from build123d import *

# Parameters (mm, degrees)
BOSS_EXTRUDE2_DEPTH = 20
SKETCH2_R           = 1.025
SKETCH2_R_2         = 1.05
SKETCH2_R_3         = 0.975
SKETCH2_R_4         = 1
SKETCH2_R_5         = 2.5
SKETCH2_R_6         = 2.55
SKETCH2_R_7         = 2.525
BOSS_EXTRUDE3_DEPTH = 20


with BuildPart() as part:
    # Sketch1 → Boss-Extrude2 (new body)
    with BuildSketch(Plane(origin=(0, 0, 0), x_dir=(1, 0, 0), z_dir=(0, 1, 0))):
        Polygon((21, -13.279056191), (21, -19.052558883), (23, -19.052558883), (23, -13.279056191), (33, -7.505553499), (43, -13.279056191), (43, -19.052558883), (45, -19.052558883), (45, -13.279056191), (55, -7.505553499), (65, -13.279056191), (65, -19.052558883), (66, -19.052558883), (66, -11.547005384), (56, -5.773502692), (56, 5.773502692), (66, 11.547005384), (66, 26.452994616), (56, 32.226497308), (56, 38), (54, 38), (54, 32.226497308), (44, 26.452994616), (34, 32.226497308), (34, 38), (32, 38), (32, 32.226497308), (22, 26.452994616), (12, 32.226497308), (12, 38), (11, 38), (11, 30.494446501), (21, 24.720943809), (21, 13.173938425), (11, 7.400435733), (11, -7.505553499), align=None)
        Polygon((12, 5.773502692), (22, 11.547005384), (32, 5.773502692), (32, -5.773502692), (22, -11.547005384), (12, -5.773502692), align=None, mode=Mode.SUBTRACT)
        Polygon((34, 5.773502692), (44, 11.547005384), (54, 5.773502692), (54, -5.773502692), (44, -11.547005384), (34, -5.773502692), align=None, mode=Mode.SUBTRACT)
        Polygon((43, 13.173938425), (33, 7.400435733), (23, 13.173938425), (23, 24.720943809), (33, 30.494446501), (43, 24.720943809), align=None, mode=Mode.SUBTRACT)
        Polygon((65, 13.173938425), (55, 7.400435733), (45, 13.173938425), (45, 24.720943809), (55, 30.494446501), (65, 24.720943809), align=None, mode=Mode.SUBTRACT)
    extrude(amount=BOSS_EXTRUDE2_DEPTH)

    # Sketch2 → Boss-Extrude3 (add, through all)
    with BuildSketch(Plane(origin=(0, 20, 0), x_dir=(1, 0, 0), z_dir=(0, 1, 0))):
        Polygon((44, 11.547005384), (34, 5.773502692), (34, -5.773502692), (44, -11.547005384), (54, -5.773502692), (54, 5.773502692), align=None)
        with Locations((44, 7.57813322)):
            Circle(SKETCH2_R, mode=Mode.SUBTRACT)
        with Locations((49.12400919, 6.50535)):
            Circle(SKETCH2_R_2, mode=Mode.SUBTRACT)
        with Locations((49.12400919, 1.82801516)):
            Circle(SKETCH2_R_3, mode=Mode.SUBTRACT)
        with Locations((38.868201604, 4.488517546)):
            Circle(SKETCH2_R_4, mode=Mode.SUBTRACT)
        with Locations((38.567822302, -1.561979816)):
            Circle(SKETCH2_R_5, mode=Mode.SUBTRACT)
        with Locations((45.13325561, -4.136659545)):
            Circle(SKETCH2_R_6, mode=Mode.SUBTRACT)
        with Locations((51.012107657, -2.763497023)):
            Circle(SKETCH2_R_7, mode=Mode.SUBTRACT)
    extrude(amount=-BOSS_EXTRUDE3_DEPTH)


solid = part.part
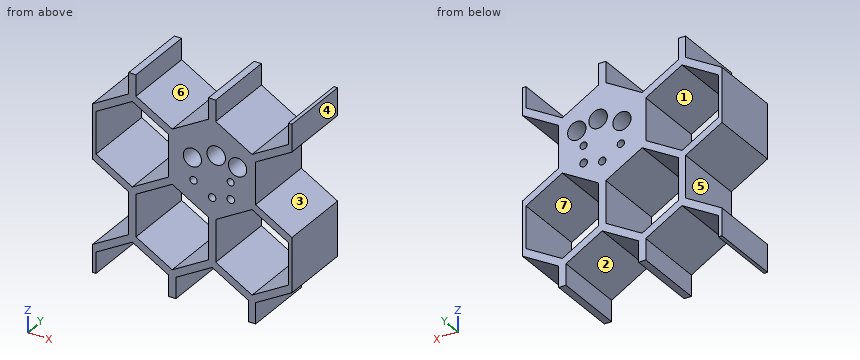
Source: CAD feature listing. Evaluate the final solid. Frame: model axes, mm. Face numbers are marked on the shaded views. A direction names the side the tool comes from. Round coordinates to 2 decimals unless told otherwise and drop trailing zeros. Loops run counter-clockwise (first coordinate to the right, second up) from the corner with the lowest first, then second, coordinate; pieces in that order, holes last. Notation, with made-up numbers: (-23, 50) - (-10, 50) arc R9 ccw to (-10, 64) - close; hole circle Ø6 at (34, 9). An arc over 180 degrees is marked (long way). Write item = value, one per line. Start each with the question number.
(1) Pin query (flat end, axial travel): pin 1 (6 mm diameter, centred on x = 33, z = -6.5, fed in from -Y); pin 2 (1 mm diameter, centred on x = 47.5, y = 13, fed in from +Z); pin 3 (1.7 mm diameter, centred on y = 13, z = 15, fed in from -X); pin 4 (6.5 mm diameter, centred on y = 14, z = -34, fed in from +X). Return the tip coordinate at first contact, or that it passes through.
(2) Section query C-C, the plane z = -10.5. Output: boundary loops of the cut face in (x, y).
(3) Set-up query: the marked faces 1, 2 and 3. Return all of +Z, -Z, +X, -X, +Y, -Y with unobstructed straight access to the full face (end or side cutting, diameter ignored); none if empty.
(4) Ray query, line 1 along X through (y, z) = (9.75, -24.5); line 2 along Z through (x, y) = (57.5, 16.25); line 3 along Z through (x, y) = (30, 8.5). Return the intervals inside material, ascending. Write a range as from..to.
(5) Section query D-D, the plane y = 2.5. State how many separate pieces and enclosed holes the cut face has, plus the area to 3 significant figures.
(6) Pull-direction query (Z, two-part tool) for the marked faces 4, 5, 6 and 7; classes: +Z half, -Z half, draft (parallel to the pull), parting line (faces both ways), or undercut.
(7) Section query B-B, the plane x = 29.5. Output: boundary loops of the cut face in (y, z).
(8) Section query A-A, the plane z = 14.5. Output: boundary loops of the cut face in (x, y), plus the area to 3 significant figures.
Conclusion:
q1.pin_1 = 0
q1.pin_2 = 12.12
q1.pin_3 = 21
q1.pin_4 = 58.56
q2.outline = (16.37, 0) - (20.19, 0) - (20.19, 20) - (16.37, 20) - close; (23.81, 0) - (27.63, 0) - (27.63, 20) - (23.81, 20) - close; (38.37, 0) - (49.63, 0) - (49.63, 20) - (38.37, 20) - close; (60.37, 0) - (64.19, 0) - (64.19, 20) - (60.37, 20) - close
q3.face_1 = +Y, -Y
q3.face_2 = -Z, +Y, -Y
q3.face_3 = +X, +Y, -Y
q4.line_1 = 21..23, 43..45, 65..66
q4.line_2 = -31.36..-29.05, -8.84..-6.64, 6.64..8.95
q4.line_3 = -31.07..-28.76, -9.13..-6.93, 6.93..9.24
q5.separate_pieces = 1
q5.enclosed_holes = 10
q5.area = 813 mm2
q6.face_4 = draft
q6.face_5 = undercut
q6.face_6 = +Z half
q6.face_7 = undercut
q7.outline = (0, -30.78) - (20, -30.78) - (20, -28.47) - (0, -28.47) - close; (0, -9.42) - (20, -9.42) - (20, -7.22) - (0, -7.22) - close; (0, 7.22) - (20, 7.22) - (20, 9.53) - (0, 9.53) - close
q8.outline = (21, 0) - (23, 0) - (23, 20) - (21, 20) - close; (43, 0) - (45, 0) - (45, 20) - (43, 20) - close; (65, 0) - (66, 0) - (66, 20) - (65, 20) - close
q8.area = 100 mm2
